The drawing under review shows one solid part. Ordinate dimensions are in mm from its lowest x, y, z. A direction names the side the tool comes from. Give positions to 0.01 mm unless a question says otherwise; leave off trailing zeros. Loops run counter-clockwise (first coordinate to the right, second up) from the corner with the lowest first, then second, coordinate; pieces in that order, holes last. Notation, with made-up numbers: M -10,35 L 38,35 A12 cw 38,45 Z; hole C -20.5,84 d3. An arc over 180 degrees is marked long. One line per item, written item: value. Start each with the question number.
Q1. Mouldability with a two-part tool opening along X and no side actions: class the marked faces 3, 4 and 5 as released by +X, released by -X, zero draft, split by the parting line, or undercut.
Q2. We need section D-D on x = 24. Write out the cut boundary in (y, z), plus the area to 3 significant figures.
Q3. We need section A-A on x = 20. Write out the cut boundary in (y, z).
Q4. To check wall thickness, follow line 1 along X through (y, z) = (22, 1); line 2 along Y through (x, z) = (7.5, 12.75); line 3 along Z through (x, y) = (5.5, 28). State the ranges of each line that lie inside material, in increasing order. Write a range as from..to.
Q5. We need section B-B on y = 21.5. Write out the cut boundary in (x, z).
Q6. For the marked faces 1 and 2, list the 3-axis set-ups (+Z, -Z, +X, -X, +Y, -Y) from which the entire face can be reached by the end or side of a thin tool; tool diameter is ignored.
Q7. For pin 1 (9 mm diameter, centred on x = 20, y = 21.5, fed in from -Z); pin 2 (8 mm diameter, centred on x = 21, z = 4.5, fed in from +Y); pin 3 (4 mm diameter, centred on y = 29, z = 4, fed in from +X), all flat-tipped, find the tip position at first contact; note any pin that passes through.
Q8. We need section C-C on z = 10. Write out the cut boundary in (x, y).
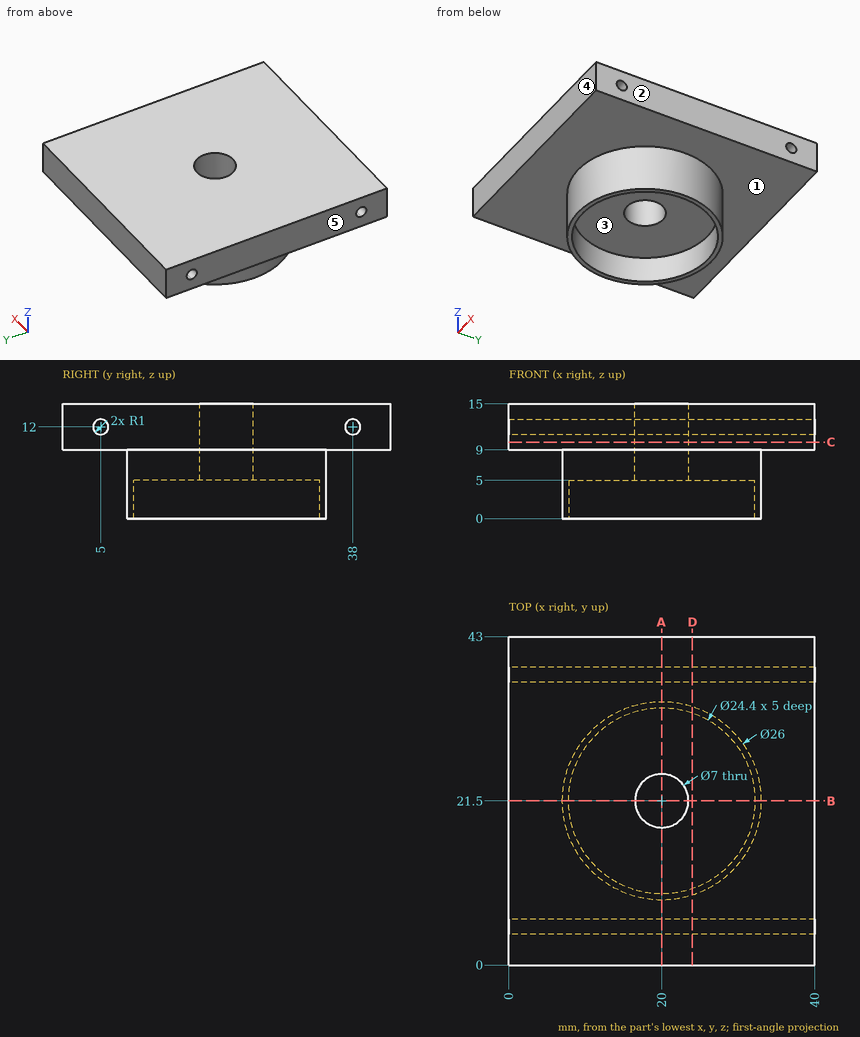
Solved:
1. face 3: undercut
1. face 4: zero draft
1. face 5: released by -X
2. outline: M 0,9 L 9.13,9 L 9.13,0 L 9.97,0 L 9.97,5 L 33.03,5 L 33.03,0 L 33.87,0 L 33.87,9 L 43,9 L 43,15 L 0,15 Z; hole C 5,12 d2; hole C 38,12 d2
2. area: 359 mm2
3. outline: M 0,9 L 8.5,9 L 8.5,0 L 9.3,0 L 9.3,5 L 18,5 L 18,15 L 0,15 Z; M 25,5 L 33.7,5 L 33.7,0 L 34.5,0 L 34.5,9 L 43,9 L 43,15 L 25,15 Z; hole C 5,12 d2; hole C 38,12 d2
4. line 1: 7.01..7.81, 32.19..32.99
4. line 2: 0..4.34, 5.66..37.34, 38.66..43
4. line 3: 9..15
5. outline: M 0,9 L 7,9 L 7,0 L 7.8,0 L 7.8,5 L 16.5,5 L 16.5,15 L 0,15 Z; M 23.5,5 L 32.2,5 L 32.2,0 L 33,0 L 33,9 L 40,9 L 40,15 L 23.5,15 Z
6. face 1: -Z
6. face 2: +Z, -Z, +X, +Y, -Y
7. pin 1: z = 5
7. pin 2: y = 34.5
7. pin 3: x = 31.78
8. outline: M 0,0 L 40,0 L 40,43 L 0,43 Z; hole C 20,21.5 d7
